```python
from build123d import *

# Parameters (mm, degrees)
SKETCH1_R       = 119.4
SKETCH1_R_2     = 114.4
EXTRUDE1_DEPTH  = 5
SKETCH2_R       = 119.4
SKETCH2_R_2     = 118.4
EXTRUDE2_DEPTH  = 5
SKETCH3_R       = 119.4
SKETCH3_R_2     = 117.4
EXTRUDE3_DEPTH  = 13
SKETCH4_R       = 117.4
SKETCH4_R_2     = 114.4
EXTRUDE4_DEPTH  = 10
EXTRUDE5_DEPTH  = 100
SKETCH6_R       = 117.4
SKETCH6_R_2     = 114.4
EXTRUDE7_DEPTH  = 15
SKETCH7_R       = 118.4
SKETCH7_R_2     = 114.4
EXTRUDE8_DEPTH  = 5
SKETCH8_R       = 117.4
SKETCH8_R_2     = 114.4
EXTRUDE9_DEPTH  = 10
EXTRUDE10_DEPTH = 270
SKETCH10_R      = 1.5
SKETCH10_R_2    = 2
EXTRUDE11_DEPTH = 3


with BuildPart() as part:
    # Sketch1 → Extrude1 (new body)
    with BuildSketch(Plane.XY):
        Circle(SKETCH1_R)
        Circle(SKETCH1_R_2, mode=Mode.SUBTRACT)
    extrude(amount=-EXTRUDE1_DEPTH)

    # Sketch2 → Extrude2 (add)
    with BuildSketch(Plane(origin=(0, 0, -5), x_dir=(-1, 0, 0), z_dir=(0, 0, -1))):
        Circle(SKETCH2_R)
        Circle(SKETCH2_R_2, mode=Mode.SUBTRACT)
    extrude(amount=EXTRUDE2_DEPTH)

    # Sketch3 → Extrude3 (add)
    with BuildSketch(Plane(origin=(0, 0, -10), x_dir=(-1, 0, 0), z_dir=(0, 0, -1))):
        Circle(SKETCH3_R)
        Circle(SKETCH3_R_2, mode=Mode.SUBTRACT)
    extrude(amount=EXTRUDE3_DEPTH)

    # Sketch4 → Extrude4 (add)
    with BuildSketch(Plane.XY):
        Circle(SKETCH4_R)
        Circle(SKETCH4_R_2, mode=Mode.SUBTRACT)
    extrude(amount=EXTRUDE4_DEPTH)

    # Sketch5 → Extrude5 (add)
    with BuildSketch(Plane.XY.offset(10)):
        with BuildLine():
            Line((20.386296, 115.61643), (19.865352, 112.662007))
            ThreePointArc((19.865352, 112.662007), (0, 114.4), (-19.865352, 112.662007))
            Line((-19.865352, 112.662007), (-20.386296, 115.61643))
            ThreePointArc((-20.386296, 115.61643), (0, 117.4), (20.386296, 115.61643))
        make_face()
        with BuildLine():
            Line((115.61643, 20.386296), (112.662007, 19.865352))
            ThreePointArc((112.662007, 19.865352), (114.4, 0), (112.662007, -19.865352))
            Line((112.662007, -19.865352), (115.61643, -20.386296))
            ThreePointArc((115.61643, -20.386296), (117.4, 0), (115.61643, 20.386296))
        make_face()
        with BuildLine():
            Line((19.865352, -112.662007), (20.386296, -115.61643))
            ThreePointArc((20.386296, -115.61643), (0, -117.4), (-20.386296, -115.61643))
            Line((-20.386296, -115.61643), (-19.865352, -112.662007))
            ThreePointArc((-19.865352, -112.662007), (0, -114.4), (19.865352, -112.662007))
        make_face()
        with BuildLine():
            Line((-112.662007, -19.865352), (-115.61643, -20.386296))
            ThreePointArc((-115.61643, -20.386296), (-117.4, 0), (-115.61643, 20.386296))
            Line((-115.61643, 20.386296), (-112.662007, 19.865352))
            ThreePointArc((-112.662007, 19.865352), (-114.4, 0), (-112.662007, -19.865352))
        make_face()
    extrude(amount=EXTRUDE5_DEPTH)

    # Sketch6 → Extrude7 (add)
    with BuildSketch(Plane.XY.offset(110)):
        Circle(SKETCH6_R)
        Circle(SKETCH6_R_2, mode=Mode.SUBTRACT)
    extrude(amount=EXTRUDE7_DEPTH)

    # Sketch7 → Extrude8 (add)
    with BuildSketch(Plane.XY.offset(125)):
        Circle(SKETCH7_R)
        Circle(SKETCH7_R_2, mode=Mode.SUBTRACT)
    extrude(amount=EXTRUDE8_DEPTH)

    # Sketch8 → Extrude9 (add)
    with BuildSketch(Plane.XY.offset(130)):
        Circle(SKETCH8_R)
        Circle(SKETCH8_R_2, mode=Mode.SUBTRACT)
    extrude(amount=EXTRUDE9_DEPTH)

    # Sketch9 → Extrude10 (add)
    with BuildSketch(Plane.XY.offset(140)):
        with BuildLine():
            Line((-20.386296, 115.61643), (-19.865352, 112.662007))
            ThreePointArc((-19.865352, 112.662007), (0, 114.4), (19.865352, 112.662007))
            Line((19.865352, 112.662007), (20.386296, 115.61643))
            ThreePointArc((20.386296, 115.61643), (0, 117.4), (-20.386296, 115.61643))
        make_face()
        with BuildLine():
            Line((112.662007, 19.865352), (115.61643, 20.386296))
            ThreePointArc((115.61643, 20.386296), (117.4, 0), (115.61643, -20.386296))
            Line((115.61643, -20.386296), (112.662007, -19.865352))
            ThreePointArc((112.662007, -19.865352), (114.4, 0), (112.662007, 19.865352))
        make_face()
        with BuildLine():
            Line((19.865352, -112.662007), (20.386296, -115.61643))
            ThreePointArc((20.386296, -115.61643), (0, -117.4), (-20.386296, -115.61643))
            Line((-20.386296, -115.61643), (-19.865352, -112.662007))
            ThreePointArc((-19.865352, -112.662007), (0, -114.4), (19.865352, -112.662007))
        make_face()
        with BuildLine():
            Line((-112.662007, -19.865352), (-115.61643, -20.386296))
            ThreePointArc((-115.61643, -20.386296), (-117.4, 0), (-115.61643, 20.386296))
            Line((-115.61643, 20.386296), (-112.662007, 19.865352))
            ThreePointArc((-112.662007, 19.865352), (-114.4, 0), (-112.662007, -19.865352))
        make_face()
    extrude(amount=EXTRUDE10_DEPTH)

    # Sketch10 → Extrude11 (add)
    with BuildSketch(Plane.XY.offset(410)):
        with BuildLine():
            Line((13.065229, 2.303752), (115.61643, 20.386296))
            ThreePointArc((115.61643, 20.386296), (117.4, 0), (115.61643, -20.386296))
            Line((115.61643, -20.386296), (13.065229, -2.303752))
            ThreePointArc((13.065229, -2.303752), (9.381031, -9.381031), (2.303752, -13.065229))
            Line((2.303752, -13.065229), (20.386296, -115.61643))
            ThreePointArc((20.386296, -115.61643), (0, -117.4), (-20.386296, -115.61643))
            Line((-20.386296, -115.61643), (-2.303752, -13.065229))
            ThreePointArc((-2.303752, -13.065229), (-9.381031, -9.381031), (-13.065229, -2.303752))
            Line((-13.065229, -2.303752), (-115.61643, -20.386296))
            ThreePointArc((-115.61643, -20.386296), (-117.4, 0), (-115.61643, 20.386296))
            Line((-115.61643, 20.386296), (-13.065229, 2.303752))
            ThreePointArc((-13.065229, 2.303752), (-9.381031, 9.381031), (-2.303752, 13.065229))
            Line((-2.303752, 13.065229), (-20.386296, 115.61643))
            ThreePointArc((-20.386296, 115.61643), (0, 117.4), (20.386296, 115.61643))
            Line((20.386296, 115.61643), (2.303752, 13.065229))
            ThreePointArc((2.303752, 13.065229), (9.381031, 9.381031), (13.065229, 2.303752))
        make_face()
        with Locations((21.92, 0)):
            Circle(SKETCH10_R, mode=Mode.SUBTRACT)
        with Locations((0, -21.92)):
            Circle(SKETCH10_R, mode=Mode.SUBTRACT)
        with Locations((-21.92, 0)):
            Circle(SKETCH10_R, mode=Mode.SUBTRACT)
        with Locations((0, 21.92)):
            Circle(SKETCH10_R, mode=Mode.SUBTRACT)
        with Locations((0, 105.043168)):
            Circle(SKETCH10_R_2, mode=Mode.SUBTRACT)
    extrude(amount=EXTRUDE11_DEPTH)


solid = part.part
```
Verification items for the finished model (mm, model axes). A direction names the side the tool comes from. Give positions to 0.01 mm unless a question says otherwise; leave off trailing zeros. Loops run counter-clockwise (first coordinate to the right, second up) from the corner with the lowest first, then second, coordinate; pieces in that order, holes last.
1. Thickness scan on line 1 (Z direction, x = -12, y = -5); line 2 (Y direction, x = -8, z = 17); line 3 (Y direction, x = 21.92, z = 410.85). Record the ranges inside material, lowest first.
2. Set-up check for faces 4 (the flat face through (27, 115, -10)), 5 (the cylindrical face through (-0.3, 117.4, 59.3)), 6 (the cylindrical face through (0.3, -117.4, 274.6)), 7 (the cylindrical face through (-117.4, -0.3, 59.3)): record each of +Z, -Z, +X, -X, +Y, -Y from which the full face is reachable in a straight line by a thin tool's end or side.
3. Section check A-A, the plane z = 206.5. Enter the section's corners in (x, y).
4. Mould release check, pull along Z, two halves, no side actions. Record for faces 1 (the flat face through (-82, -82, 140)), 2 (the cylindrical face through (117.4, 0.3, 274.6)), 3 (the cylindrical face through (111.98, 35.26, 4.93)): released by +Z, released by -Z, zero draft, split by the parting line, or undercut.
5. Section check B-B, the plane y = 96.5. Count the separate pieces of the cut face and the enclosed holes in it, then the cut area to 3 significant figures.
6. Go/stop test with flat-tipped pins: pin 1 Ø8 at (x, z) = (-15, 135.5) entering from -Y; pin 2 Ø2.5 at (x, y) = (0, -21.92) entering from +Z; pin 3 Ø4 at (x, y) = (0, 21.92) entering from -Z; pin 4 Ø10 at (y, z) = (-58.5, 143) entering from +X. Record where each tip stops, or that it passes through.
Geometry says:
1. line 1: z = 410 to 413
1. line 2: y = -117.13 to -114.12, 114.12 to 117.13
1. line 3: y = -3.87 to -1.5, 1.5 to 3.87
2. face 4: none
2. face 5: +Y
2. face 6: +Z, -Y
2. face 7: -X
3. outline: (-115.62, -20.39) - (-112.66, -19.87) arc R114.4 cw to (-112.66, 19.87) - (-115.62, 20.39) arc R117.4 ccw to start; (-20.39, -115.62) arc R117.4 ccw to (20.39, -115.62) - (19.87, -112.66) arc R114.4 cw to (-19.87, -112.66) - close; (-20.39, 115.62) - (-19.87, 112.66) arc R114.4 cw to (19.87, 112.66) - (20.39, 115.62) arc R117.4 ccw to start; (112.66, -19.87) - (115.62, -20.39) arc R117.4 ccw to (115.62, 20.39) - (112.66, 19.87) arc R114.4 cw to start
4. face 1: released by +Z
4. face 2: zero draft
4. face 3: undercut
5. separate pieces: 5
5. enclosed holes: 0
5. area: 749 mm2
6. pin 1: stops at y = -116.88
6. pin 2: passes through
6. pin 3: stops at z = 410
6. pin 4: stops at x = 103.98
